CAD build for the part. Positions are in the model's coordinates, mm. A direction names the side the tool comes from. Coordinates: 2 decimals unless noted, no trailing zeros. Loops run counter-clockwise (first coordinate to the right, second up) from the corner with the lowest first, then second, coordinate; pieces in that order, holes last.
1) Saw through at D-D, the plane y = -34. Write the cut outline in (x, z).
2) Wall check: line 1 along Y through (x, z) = (-7, 5.05); line 2 along X through (y, z) = (-10, 0.3); line 3 along Y through (x, z) = (15, 0.3). Give the ranges that are in metal, low to high.
3) Saw through at C-C, the plane x = 15. Write the cut outline in (y, z).
4) Two-plate mould, pull along X, no slides. Class faces 1 (the flat face through (5.434, -44.606, 2.958)), 2 (the flat face through (-20, -48, 3)), 3 (the flat face through (0, -48, 3)), 4 (the flat face through (15, 2, 3)): +X half, -X half, draft (parallel to the pull), parting line (faces both ways), or undercut.
5) Which spindle directions (+Z, -Z, +X, -X, +Y, -Y) get a long thin tool onto all of the face, cutting with end or side? Do faces 5 (the flat face through (-13.3, 1, 3)), 6 (the flat face through (-3, -49, 3)), 7 (the flat face through (16.7, 1, 3)), 8 (the flat face through (-5.434, -44.606, 2.958)). Say none if no direction does.
6) Saw through at A-A, the plane x = -8. Write the cut outline in (y, z), and give its area (3 significant figures).
7) Pin check, flat tips, straight feed: pin 1 Ø3 at (x, z) = (0.5, 2) entering from +Y; pin 2 Ø1.8 at (y, z) = (-23.5, 4) entering from -X; pin 3 Ø1 at (y, z) = (-11.5, 5) entering from +X. Stop position of each tip, or through.
```python
from build123d import *

# Parameters (mm, degrees)
F1_DEPTH = 6
F3_DEPTH = 6
F4_SIZE  = 0.2


with BuildPart() as f1:
    # F0 (on Top) → F1 (new body)
    with BuildSketch(Plane.XY):
        Polygon((6.828427, -46), (4, -43.171573), (4, -46), align=None)
        Polygon((20, 0), (0, 0), (0, -48), (3, -48), (3, -50), (20, -50), (20, -46), (16, -46), (6.828427, -46), (4, -46), (4, -43.171573), (4, -4), (16, -4), (20, -4), align=None)
    extrude(amount=F1_DEPTH)

    # F2 (on Top) → F3 (join, through all)
    with BuildSketch(Plane.XY):
        Polygon((14.3, 0), (15.7, 0), (17.7, 2), (12.3, 2), align=None)
    extrude(amount=F3_DEPTH)

    # F4
    f4_edges = [f1.edges().sort_by_distance(p)[0] for p in [
        (17.7, 2, 3),
        (12.3, 2, 3),
        (15.7, 0, 3),
        (14.3, 0, 3),
    ]]
    chamfer(f4_edges, length=F4_SIZE)

    # F5: F1 across face


with BuildPart() as f1_1:
    add(f1.part)
    add(f1.part.mirror(Plane(origin=(0, -24, 3), x_dir=(0, -1, 0), z_dir=(-1, 0, 0))))


solid = f1_1.part
```
Data:
1. outline: (-4, 0) - (4, 0) - (4, 6) - (-4, 6) - close
2. line 1: y = -50 to -46, -4 to 0
2. line 2: x = -4 to 4
2. line 3: y = -50 to -46, -4 to 2
3. outline: (-50, 0) - (-46, 0) - (-46, 6) - (-50, 6) - close; (-4, 0) - (2, 0) - (2, 6) - (-4, 6) - close
4. face 1: +X half
4. face 2: -X half
4. face 3: undercut
4. face 4: draft
5. face 5: +Z, -Z
5. face 6: +Z, -Z, -Y
5. face 7: +Z, -Z, +X
5. face 8: +Z, -Z, -X
6. outline: (-50, 0) - (-46, 0) - (-46, 6) - (-50, 6) - close; (-4, 0) - (0, 0) - (0, 6) - (-4, 6) - close
6. area: 48.0 mm2
7. pin 1: stops at y = 0
7. pin 2: stops at x = -4
7. pin 3: stops at x = 4
